Input: part model. Units: mm. Frame: model coordinates. Face numbers are marked on the shaded views. A direction names the side the tool comes from. Give positions to 0.01 mm unless a question says otherwise; leave off trailing zeros. Order: outer loops, then holes, each group sorted by start corner. A loop starts at its lowest first (then second) coordinate and runs counter-clockwise, first axis right, second up. Notation, with made-up numbers: (35, 75.25) - (67, 75.25) arc R22 ccw to (67, 84.25) - close; hole circle Ø5 at (36.5, 77.5). An arc over 180 degrees is marked (long way). Answer in a Markdown table with one row per item. Add a question column.
1. Ray query, line 1 (Z direction, x = -19, y = 1.5); line 2 (Z direction, x = -5, y = -4.75) (3 decimals); line 3 (Z direction, x = -5, y = 2.5) (3 decimals). Return the intervals inside material, ascending. Write a range as [from, to].
2. Contact query for flat-ended pins moving along their axis: pin 1 (5 mm diameter, centred on x = -17, z = -31.55, fed in from +Y); pin 2 (3.5 mm diameter, centred on x = 19, z = -14.55, fed in from -Y); pin 3 (6.5 mm diameter, centred on y = 4.5, z = 21, fed in from -X). Output: stop coordinate, or through.
3. Section query A-A on z = 4. Return loops of the section in (x, y).
4. Section query B-B on x = 35. Return loops of the section in (y, z), and give its area (3 significant figures).
5. Access query for the marked faces 1, 2 and 3. Directions: +Z, -Z, +X, -X, +Y, -Y. A direction counts if a zero-diameter tool reaches every point of the face in a straight line with its end or side. Return the directions, or none.
6. Section query D-D on y = 3.75. Count the separate pieces of the cut face and the enclosed holes in it, and give its area (3 significant figures).
7. Mould query, pull axis Y, two halves, no side actions, for the marked faces 4, 5 and 6. Classes: released by +Y, released by -Y, zero draft, split by the parting line, or undercut.
8. Section query C-C on x = -5. Return loops of the section in (y, z) (3 decimals), and give its area (3 significant figures).
```python
from build123d import *

# Parameters (mm, degrees)
MAIN_BODY_DEPTH           = 10
SKETCH2_R                 = 2.325
SKETCH2_R_2               = 2.05
SKETCH2_W                 = 21.5
SKETCH2_H                 = 42.4
SERVO_ROTROD_CUTOUT_DEPTH = 30
SKETCH3_W                 = 18
SKETCH3_H                 = 8
SERVO_CABLE_CUTOUT_DEPTH  = 57.102305
CONTROL_ARM_CUTOUT_START  = -66
SKETCH4_W                 = 24.86969785
SKETCH4_H                 = 10
CONTROL_ARM_CUTOUT_DEPTH  = 67
FILLET1_R                 = 4
SKETCH6_R                 = 1.6
MOUNT_HOLES_CHASSIS_DEPTH = 21
SKETCH7_R                 = 3.25
BOLT_HEAD_HOLES_DEPTH     = 4.5


with BuildPart() as part:
    # Sketch1 → Main-Body (new body, symmetric)
    with BuildSketch(Plane(origin=(0, 0, 0), x_dir=(1, 0, 0), z_dir=(0, 1, 0))):
        Polygon((20, 39.547694656), (-20, 39.547694656), (-25.13030215, 25.452305344), (-50, 10), (-50, -10), (-25.13030215, -25.452305344), (25.13030215, -25.452305344), (50, -10), (50, 10), (25.13030215, 25.452305344), align=None)
    extrude(amount=MAIN_BODY_DEPTH, both=True)

    # Sketch2 → Servo&RotRod-Cutout (cut)
    with BuildSketch(Plane(origin=(0, 10, 0), x_dir=(1, 0, 0), z_dir=(0, 1, 0))):
        with Locations((-5, -13.5)):
            Circle(SKETCH2_R)
        with Locations((5, -13.5)):
            Circle(SKETCH2_R)
        with Locations((-5, 34.4)):
            Circle(SKETCH2_R)
        with Locations((5, 34.4)):
            Circle(SKETCH2_R)
        with Locations((-42, 0)):
            Circle(SKETCH2_R_2)
        with Locations((42, 0)):
            Circle(SKETCH2_R_2)
        with Locations((0, 10.45)):
            Rectangle(SKETCH2_W, SKETCH2_H)
    extrude(amount=-SERVO_ROTROD_CUTOUT_DEPTH, mode=Mode.SUBTRACT)

    # Sketch3 → Servo-Cable-Cutout (cut)
    with BuildSketch(Plane.XY.offset(25.452305344)):
        with Locations((0, 6)):
            Rectangle(SKETCH3_W, SKETCH3_H)
    extrude(amount=-SERVO_CABLE_CUTOUT_DEPTH, mode=Mode.SUBTRACT)

    # Sketch4 → Control-Arm-Cutout (cut)
    with BuildSketch(Plane.XY.offset(25.452305344).offset(CONTROL_ARM_CUTOUT_START)):
        with Locations((-37.565151075, 0)):
            Rectangle(SKETCH4_W, SKETCH4_H)
    control_arm_cutout = extrude(amount=CONTROL_ARM_CUTOUT_DEPTH, mode=Mode.SUBTRACT)

    # Mirror1: Control-Arm-Cutout across plane
    add(control_arm_cutout.mirror(Plane(origin=(0, 0, 0), x_dir=(0, 0, 1), z_dir=(1, 0, 0))), mode=Mode.SUBTRACT)

    # Fillet1
    fillet1_edges = [part.edges().sort_by_distance(p)[0] for p in [
        (-25.13030215, 5, 0),
        (-25.13030215, -5, 0),
        (25.13030215, -5, 0),
        (25.13030215, 5, 0),
    ]]
    fillet(fillet1_edges, radius=FILLET1_R)

    # Sketch6 → Mount-Holes-Chassis (cut, through all)
    with BuildSketch(Plane.XZ.offset(10)):
        with Locations((19, -14.547694656)):
            Circle(SKETCH6_R)
        with Locations((19, 13.452305344)):
            Circle(SKETCH6_R)
        with Locations((17, -31.547694656)):
            Circle(SKETCH6_R)
        with Locations((-17, -31.547694656)):
            Circle(SKETCH6_R)
        with Locations((-19, 13.452305344)):
            Circle(SKETCH6_R)
        with Locations((-19, -14.547694656)):
            Circle(SKETCH6_R)
    extrude(amount=-MOUNT_HOLES_CHASSIS_DEPTH, mode=Mode.SUBTRACT)

    # Sketch7 → Bolt-Head-Holes (cut)
    with BuildSketch(Plane.XZ.offset(10)):
        with Locations((17, -31.547694656)):
            Circle(SKETCH7_R)
        with Locations((19, -14.547694656)):
            Circle(SKETCH7_R)
        with Locations((19, 13.452305344)):
            Circle(SKETCH7_R)
        with Locations((-19, 13.452305344)):
            Circle(SKETCH7_R)
        with Locations((-19, -14.547694656)):
            Circle(SKETCH7_R)
        with Locations((-17, -31.547694656)):
            Circle(SKETCH7_R)
    extrude(amount=-BOLT_HEAD_HOLES_DEPTH, mode=Mode.SUBTRACT)


solid = part.part
```
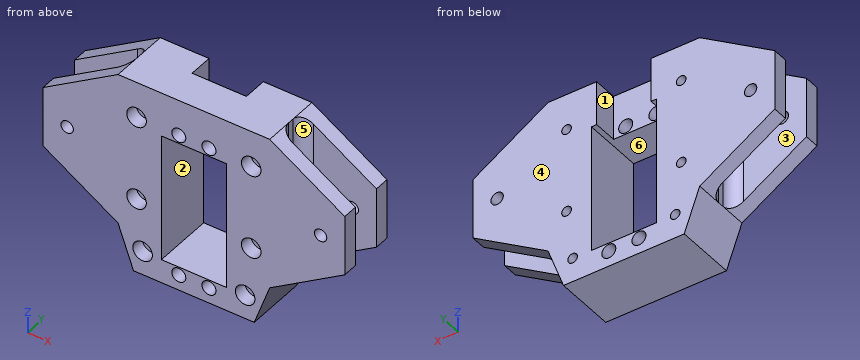
Answer:
| question | item | result |
|---|---|---|
| 1 | line 1 | z = [-39.55, -16.15], [-12.95, 11.85], [15.05, 25.45] |
| 1 | line 2 | z = [-39.548, -36.725], [-32.075, -31.65], [10.75, 11.175], [15.825, 25.452] |
| 1 | line 3 | z = [-39.548, -36.725], [-32.075, -31.65] |
| 2 | pin 1 | stops at y = 10 |
| 2 | pin 2 | stops at y = -5.5 |
| 2 | pin 3 | stops at x = -37.46 |
| 3 | outline | (-50, -10) - (-10.75, -10) - (-10.75, 10) - (-50, 10) - (-50, 5) - (-29.13, 5) arc R4 cw to (-25.13, 1) - (-25.13, -1) arc R4 cw to (-29.13, -5) - (-50, -5) - close; (10.75, -10) - (50, -10) - (50, -5) - (29.13, -5) arc R4 cw to (25.13, -1) - (25.13, 1) arc R4 cw to (29.13, 5) - (50, 5) - (50, 10) - (10.75, 10) - close |
| 4 | outline | (-10, -19.32) - (-5, -19.32) - (-5, 19.32) - (-10, 19.32) - close; (5, -19.32) - (10, -19.32) - (10, 19.32) - (5, 19.32) - close |
| 4 | area | 386 mm² |
| 5 | face 1 | +Z, +Y |
| 5 | face 2 | +Y, -Y |
| 5 | face 3 | +Z, -Z, -X |
| 6 | separate pieces | 1 |
| 6 | enclosed holes | 8 |
| 6 | area | 2,050 mm² |
| 7 | face 4 | released by +Y |
| 7 | face 5 | undercut |
| 7 | face 6 | zero draft |
| 8 | outline | (-10, -39.548) - (10, -39.548) - (10, -36.725) - (-10, -36.725) - close; (-10, -32.075) - (10, -32.075) - (10, -31.65) - (-10, -31.65) - close; (-10, 10.75) - (2, 10.75) - (2, 11.175) - (-10, 11.175) - close; (-10, 15.825) - (2, 15.825) - (2, 25.452) - (-10, 25.452) - close |
| 8 | area | 186 mm² |
